Part model, mm, in its own coordinate system. A direction names the side the tool comes from. Round coordinates to 2 decimals unless told otherwise and drop trailing zeros. Write each loop counter-clockwise with the first axis right and the second up, starting at its lowest first coordinate (ties: lowest second). Pieces come first, ordered by that corner, then holes. Notation, with made-up numbers: (-25.5, 80) -> (-2.5, 80) arc R24 ccw to (-2.5, 111) -> close; hole circle Ø11 at (35, 47). An arc over 180 degrees is marked (long way). Return JSON: item names as keys, results as strings. Group by question number.
(1) Tool access for faces 1 (the flat face through (-7.2, 9, 16.764)), 2 (the flat face through (0, 1, 0)): list every direction of +Z, -Z, +X, -X, +Y, -Y with a clear straight run to the whole face (end or side of a thin tool).
(2) Saw through at C-C (z = 19). List the corners of the cut face in (x, y).
(3) Saw through at A-A (y = 0). List the corners of the cut face in (x, z).
(4) Drop flat-ended pins along their axis: pin 1 Ø10 at (x, y) = (16, 5.5) entering from +Z; pin 2 Ø6 at (y, z) = (17.5, 21.5) entering from +X. Give the stop position or say it passes through.
(5) Saw through at B-B (x = -1). List the corners of the cut face in (y, z).
(6) Saw through at D-D (y = 10). List the corners of the cut face in (x, z).
(7) Drill centre lines: L1, parallel to Z at x = 7, y = -32; L2, parallel to X at y = -4.5, z = 17; L3, parallel to Y at x = -8, z = 29. Where is each one in solid material? Low to high. Write a range as from..to.
from build123d import *

# Parameters (mm, degrees)
F0_W          = 61.2063445151
F0_H          = 75.9055092931
F1_DEPTH      = 16.764
F2_R          = 11.3569479506
F3_DEPTH      = 15.748
F5_DEPTH      = 25.4
F5_DEPTH_BACK = 25.4


with BuildPart() as f1:
    # F0 (on Top) → F1 (new body)
    with BuildSketch(Plane.XY):
        Rectangle(F0_W, F0_H)
    extrude(amount=F1_DEPTH)

    # F2 (on face) → F3 (join)
    with BuildSketch(Plane.XY.offset(16.764)):
        Circle(F2_R)
    extrude(amount=F3_DEPTH)

    # F4 (on Front) → F5 (cut, two sides)
    with BuildSketch(Plane.XZ) as f5_sk:
        Polygon((12.6237450168, 32.6778665185), (-11.2310564145, 32.6778665185), (12.6237450168, 22.2839899361), align=None)
    extrude(amount=-F5_DEPTH, mode=Mode.SUBTRACT)
    extrude(f5_sk.sketch, amount=F5_DEPTH_BACK, mode=Mode.SUBTRACT)


solid = f1.part
Computed values:
{
 "1": {"face 1": "+Z", "face 2": "-Z, +X, -X, +Y, -Y"},
 "2": {"outline": "circle Ø22.71 at (0, 0)"},
 "3": {"outline": "(-30.6, 0) -> (30.6, 0) -> (30.6, 16.76) -> (11.36, 16.76) -> (11.36, 22.84) -> (-10.85, 32.51) -> (-11.36, 32.51) -> (-11.36, 16.76) -> (-30.6, 16.76) -> close"},
 "4": {"pin 1": "z = 16.76", "pin 2": "through"},
 "5": {"outline": "(-37.95, 0) -> (37.95, 0) -> (37.95, 16.76) -> (11.31, 16.76) -> (11.31, 28.22) -> (-11.31, 28.22) -> (-11.31, 16.76) -> (-37.95, 16.76) -> close"},
 "6": {"outline": "(-30.6, 0) -> (30.6, 0) -> (30.6, 16.76) -> (5.38, 16.76) -> (5.38, 25.44) -> (-5.38, 30.13) -> (-5.38, 16.76) -> (-30.6, 16.76) -> close"},
 "7": {"L1": "0..16.76", "L2": "-10.43..10.43", "L3": "-8.06..8.06"}
}
